Here's how the part is built. I have some questions about the finished solid (model axes, mm). Face numbers are marked on the shaded views. A direction names the side the tool comes from. Round coordinates to 2 decimals unless told otherwise and drop trailing zeros. Write each loop counter-clockwise with the first axis right and the second up, starting at its lowest first coordinate (ties: lowest second). Pieces come first, ordered by that corner, then holes. Notation, with made-up numbers: (-6.75, 19.5) -> (39.25, 19.5) arc R37 cw to (39.25, 58.5) -> close; hole circle Ø1 at (-20.75, -15.75). An arc over 180 degrees is marked (long way). Answer in a Markdown table with one row per item. Add a question column.
from build123d import *

# Parameters (mm, degrees)
EXTRUDE_1_DEPTH          = 15
SKETCH_9_W               = 10
SKETCH_9_H               = 33
SKETCH_12_W              = 10
SKETCH_12_H              = 28
FILLET_1_R               = 5
EXTRUDE_4_DEPTH          = 8
SKETCH_17_R              = 7
CUT_EXTRUDE_1_DEPTH      = 5
CUT_EXTRUDE_2_DEPTH      = 75.692703794
CUT_EXTRUDE_2_DEPTH_BACK = 75.692703794
SKETCH_18_R              = 4


with BuildPart() as part:
    # 草图1 → 凸台-拉伸1 (new body)
    with BuildSketch(Plane(origin=(0, 0, 0), x_dir=(1, 0, 0), z_dir=(0, 1, 0))):
        with BuildLine():
            Line((-31.622776602, 45), (31.622776602, 45))
            ThreePointArc((31.622776602, 45), (55, 0), (31.622776602, -45))
            Line((31.622776602, -45), (-31.622776602, -45))
            ThreePointArc((-31.622776602, -45), (-55, 0), (-31.622776602, 45))
        make_face()
    extrude(amount=EXTRUDE_1_DEPTH)

    # 草图9 → 旋转1 (revolve)
    with BuildSketch(Plane.XY, mode=Mode.PRIVATE) as revolve_1_sk:
        Polygon((20, 33), (20, 43), (10, 33), align=None)
        with Locations((15, 16.5)):
            Rectangle(SKETCH_9_W, SKETCH_9_H)
    revolve(revolve_1_sk.sketch.rotate(Axis((0, 0, 0), (0, 1, 0)), 90), axis=Axis((0, 0, 0), (0, 1, 0)))

    # 草图12 → 旋转2 (revolve)
    with BuildSketch(Plane.XY, mode=Mode.PRIVATE) as revolve_2_sk:
        with Locations((25, 29)):
            Rectangle(SKETCH_12_W, SKETCH_12_H)
    revolve(revolve_2_sk.sketch.rotate(Axis((0, 0, 0), (0, 1, 0)), 90), axis=Axis((0, 0, 0), (0, 1, 0)))

    # 圆角1
    fillet_1_edges = [part.edges().sort_by_distance(p)[0] for p in [
        (0, 43, 20),
        (0, 43, 30),
    ]]
    fillet(fillet_1_edges, radius=FILLET_1_R)

    # 草图14 → 凸台-拉伸4 (add)
    with BuildSketch(Plane(origin=(0, 15, 0), x_dir=(1, 0, 0), z_dir=(0, 1, 0))):
        with BuildLine():
            Line((-27.037011669, 13), (-40, 13))
            ThreePointArc((-40, 13), (-53, 0), (-40, -13))
            Line((-40, -13), (-27.037011669, -13))
            ThreePointArc((-27.037011669, -13), (-29.249874787, -6.666695205), (-30, 0))
            ThreePointArc((-30, 0), (-29.249874787, 6.666695205), (-27.037011669, 13))
        make_face()
        with BuildLine():
            Line((27.037011669, -13), (40, -13))
            ThreePointArc((40, -13), (53, 0), (40, 13))
            Line((40, 13), (27.037011669, 13))
            ThreePointArc((27.037011669, 13), (30, 0), (27.037011669, -13))
        make_face()
    extrude(amount=EXTRUDE_4_DEPTH)

    # 草图17 → 切除-拉伸1 (cut)
    with BuildSketch(Plane(origin=(0, 23, 0), x_dir=(1, 0, 0), z_dir=(0, 1, 0))):
        with Locations(Location((-40, 0, 0), (0, 0, 270))):
            Circle(SKETCH_17_R)
        with Locations(Location((40, 0, 0), (0, 0, 270))):
            Circle(SKETCH_17_R)
    extrude(amount=-CUT_EXTRUDE_1_DEPTH, mode=Mode.SUBTRACT)

    # 草图18 → 切除-拉伸2 (cut, two sides: drawn at the far end of the back side and taken through both)
    with BuildSketch(Plane(origin=(0, 23, 0), x_dir=(1, 0, 0), z_dir=(0, 1, 0)).offset(-CUT_EXTRUDE_2_DEPTH_BACK)):
        with Locations(Location((-40, 0, 0), (0, 0, 270))):
            Circle(SKETCH_18_R)
        with Locations(Location((40, 0, 0), (0, 0, 270))):
            Circle(SKETCH_18_R)
    extrude(amount=CUT_EXTRUDE_2_DEPTH + CUT_EXTRUDE_2_DEPTH_BACK, mode=Mode.SUBTRACT)


solid = part.part
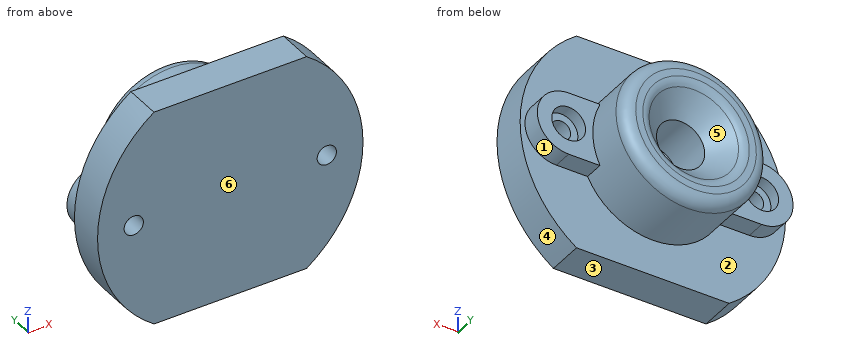
Item 1: If we section it at B-B on x = 0: Please give me the cut outline in (y, z).
Item 2: For P1, Ø8.5, axis at x = 40, z = 0, coming from the +Y side; P2, Ø2.5, axis at x = -31.5, y = 19.5, coming from the -Z side; P3, Ø3, axis at x = -13, y = 32.5, coming from the +Z side, each with a flat end and sliding along its axis, tell me the tip position at first contact or that it passes through.
Item 3: If we section it at A-A on y = 11: Please give me the cut outline in (x, z), then the cut area to 3 significant figures.
Item 4: If we section it at C-C on z = 0: Give the number of separate pieces and of enclosed holes in the cut face, then the cut area to 3 significant figures.
Item 5: If we mould it in two halves opening along X, with no side actions, what happens to the marked faces 4, 5 and 6? For each: pulls with the +X half, pulls with the -X half, needs draft (parallel to the pull), parting line crosses it, or undercut.
Item 6: I need wall thicknesses on line 1 along X through (y, z) = (22, 0); line 2 along Y through (x, z) = (42.5, 14.5); line 3 along Z through (x, y) = (40, 3.5). Which ranges of each line are inside material? Lowest first, please. Write a range as from..to.
Item 7: On a 3-axis mill with a long thin cutter (end or side, diameter ignored), from which of +Z, -Z, +X, -X, +Y, -Y can I reach the whole of each face in a straight line? I mean the marked faces 1, 2 and 3. Say none if no direction works.
Results list:
| question | item | result |
|---|---|---|
| 1 | outline | (0, -45) -> (15, -45) -> (15, -30) -> (38, -30) arc R5 ccw to (43, -25) -> (43, -22.07) arc R5 ccw to (41.54, -18.54) -> (33, -10) -> (15, -10) -> (15, 10) -> (33, 10) -> (41.54, 18.54) arc R5 ccw to (43, 22.07) -> (43, 25) arc R5 ccw to (38, 30) -> (15, 30) -> (15, 45) -> (0, 45) -> close |
| 2 | P1 | y = 18 |
| 2 | P2 | z = -13 |
| 2 | P3 | z = 27.71 |
| 3 | outline | (-31.62, -45) -> (31.62, -45) arc R55 ccw to (31.62, 45) -> (-31.62, 45) arc R55 ccw to start; hole circle Ø8 at (-40, 0); hole circle Ø8 at (40, 0) |
| 3 | area | 8,540 mm² |
| 4 | separate pieces | 3 |
| 4 | enclosed holes | 0 |
| 4 | area | 2,600 mm² |
| 5 | face 4 | pulls with the +X half |
| 5 | face 5 | undercut |
| 5 | face 6 | needs draft |
| 6 | line 1 | -53..-47, -33..-10, 10..33, 47..53 |
| 6 | line 2 | 0..15 |
| 6 | line 3 | -37.75..-4, 4..37.75 |
| 7 | face 1 | +X, +Y |
| 7 | face 2 | +Y |
| 7 | face 3 | -Z, +X, -X, +Y, -Y |
